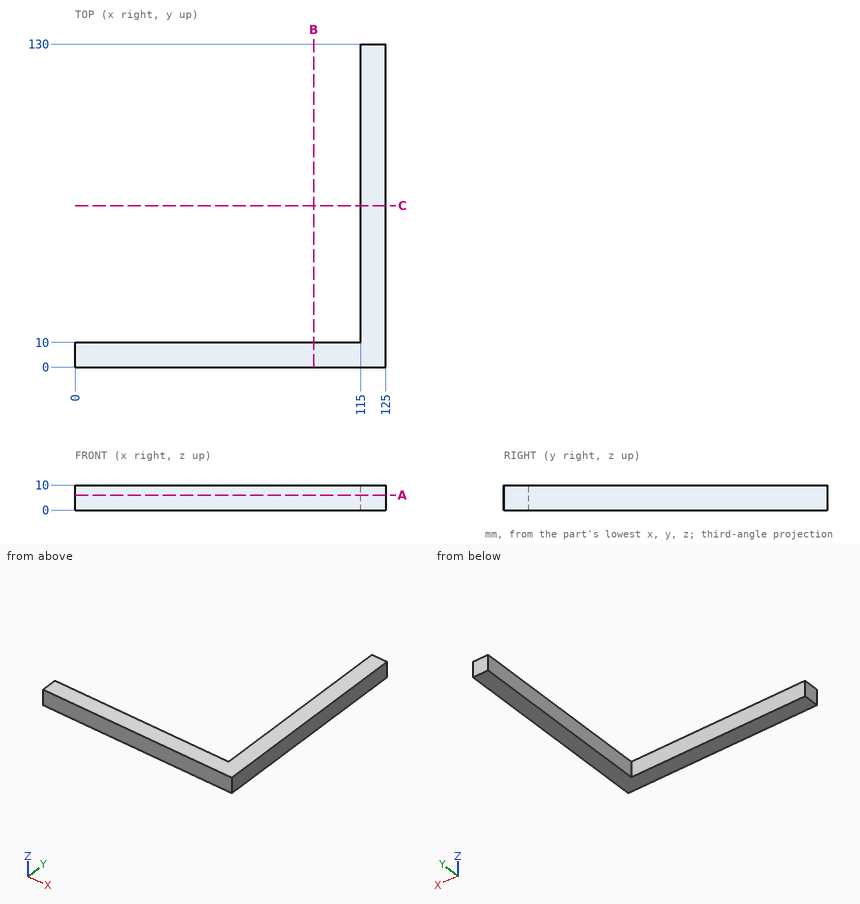
The drawing under review shows one solid part. Ordinate dimensions are in mm from its lowest x, y, z. Coordinates: 2 decimals unless noted, no trailing zeros. Order: outer loops, then holes, each group sorted by start corner. A loop starts at its lowest first (then second) coordinate and runs counter-clockwise, first axis right, second up. Notation, with made-up numbers: (-10, -18) -> (10, -18) arc R32 ccw to (10, 17) -> close; hole circle Ø6 at (-25, -12.75). An arc over 180 degrees is marked (long way). Use CSV: the item, a comma, the result in double quotes. Start each with the question number.
Item 1: We need section B-B, the plane x = 96. Give the boundary of the cut face in (y, z), then the cut area to 3 significant figures.
Item 2: Wall thickness on probe 1 along X at (y, z) = (56.5, 5.75); probe 2 along Y at (x, z) = (78, 8.75): over which ranges is each line inside the solid? List them lowest first.
Item 3: We need section A-A, the plane z = 6. Give the boundary of the cut face in (x, y).
Item 4: We need section C-C, the plane y = 65. Give the boundary of the cut face in (x, z), then the cut area to 3 significant figures.
Item 5: Insertion check: pin 1 (5 mm diameter, centred on y = 63.5, z = 3.5, fed in from -X). The pin has a flat end and moves straight along its axis. Give the tip position at first contact, or say it passes through.
Derived:
1,outline,"(0, 0) -> (10, 0) -> (10, 10) -> (0, 10) -> close"
1,area,"100 mm^2"
2,probe 1,"x = 115 to 125"
2,probe 2,"y = 0 to 10"
3,outline,"(0, 0) -> (125, 0) -> (125, 130) -> (115, 130) -> (115, 10) -> (0, 10) -> close"
4,outline,"(115, 0) -> (125, 0) -> (125, 10) -> (115, 10) -> close"
4,area,"100 mm^2"
5,pin 1,"stops at x = 115"
